Source: CAD feature listing. Evaluate the final solid. Frame: model axes, mm. A direction names the side the tool comes from. Give positions to 0.01 mm unless a question says otherwise; leave off trailing zeros. Loops run counter-clockwise (first coordinate to the right, second up) from the corner with the lowest first, then second, coordinate; pieces in that order, holes last. Notation, with made-up numbers: M -30.5,62.25 L -13.5,62.25 A35 cw -13.5,97.25 Z; hole C 67,14 d10. An arc over 180 degrees is marked long. Answer in a Markdown table with one row per item.
```python
from build123d import *

# Parameters (mm, degrees)
CROQUIS1_R              = 1.000000216
CROQUIS1_R_2            = 1.000000063
CROQUIS1_R_3            = 1.000000073
CROQUIS1_R_4            = 0.999999979
CROQUIS1_R_5            = 1.000000424
CROQUIS1_R_6            = 1.000000593
CROQUIS1_W              = 42
CROQUIS1_H              = 20
SALIENTE_EXTRUIR1_DEPTH = 5.5
CROQUIS2_W              = 16.5
CROQUIS2_H              = 2.5
SALIENTE_EXTRUIR2_DEPTH = 0.5
CROQUIS3_W              = 16.5
CROQUIS3_H              = 20
CORTAR_EXTRUIR1_DEPTH   = 2.5
REDONDEO1_R             = 3


with BuildPart() as part:
    # Croquis1 → Saliente-Extruir1 (new body)
    with BuildSketch(Plane(origin=(0, 0, 0), x_dir=(1, 0, 0), z_dir=(0, 1, 0))):
        with BuildLine():
            Line((-35.503347099, 12.623865495), (-35.503347099, 5.124115358))
            Line((-35.503347099, 5.124115358), (-25.50434655, 7.623865495))
            Line((-25.50434655, 7.623865495), (-25.50434655, -7.376134505))
            Line((-25.50434655, -7.376134505), (-35.503347099, -4.876384368))
            Line((-35.503347099, -4.876384368), (-35.503347099, -12.376134505))
            Line((-35.503347099, -12.376134505), (-19.003347099, -12.376134505))
            Line((-19.003347099, -12.376134505), (-12.8396222, -15.276134123))
            Line((-12.8396222, -15.276134123), (34.184025109, -15.270214667))
            ThreePointArc((34.184025109, -15.270214667), (36.167856769, -14.448338396), (36.98973304, -12.464506735))
            Line((36.98973304, -12.464506735), (36.98973304, 12.712237726))
            ThreePointArc((36.98973304, 12.712237726), (36.167960213, 14.69617283), (34.184025109, 15.517945657))
            Line((34.184025109, 15.517945657), (-12.8396222, 15.523865114))
            Line((-12.8396222, 15.523865114), (-19.003347099, 12.623865495))
            Line((-19.003347099, 12.623865495), (-35.503347099, 12.623865495))
        make_face()
        with Locations((-22.254346372, 6.123865279)):
            Circle(CROQUIS1_R, mode=Mode.SUBTRACT)
        with Locations((-15.504346839, 5.123865558)):
            Circle(CROQUIS1_R_2, mode=Mode.SUBTRACT)
        with Locations((33.495653377, 5.123865568)):
            Circle(CROQUIS1_R_3, mode=Mode.SUBTRACT)
        with Locations((33.4956531, -4.876133997)):
            Circle(CROQUIS1_R_4, mode=Mode.SUBTRACT)
        with Locations((-15.504347678, -4.876134927)):
            Circle(CROQUIS1_R_5, mode=Mode.SUBTRACT)
        with Locations((-22.254345484, -5.876135091)):
            Circle(CROQUIS1_R_6, mode=Mode.SUBTRACT)
        with Locations((8.99565345, 0.123865495)):
            Rectangle(CROQUIS1_W, CROQUIS1_H, mode=Mode.SUBTRACT)
    extrude(amount=SALIENTE_EXTRUIR1_DEPTH)

    # Croquis2 → Saliente-Extruir2 (add)
    with BuildSketch(Plane(origin=(0, 5.5, 0), x_dir=(1, 0, 0), z_dir=(0, 1, 0))):
        with Locations((-27.253347099, -11.126134505)):
            Rectangle(CROQUIS2_W, CROQUIS2_H)
        with Locations((-27.253347099, 11.373865495)):
            Rectangle(CROQUIS2_W, CROQUIS2_H)
    extrude(amount=SALIENTE_EXTRUIR2_DEPTH)

    # Croquis3 → Cortar-Extruir1 (cut)
    with BuildSketch(Plane(origin=(0, 5.5, 0), x_dir=(1, 0, 0), z_dir=(0, 1, 0))):
        with Locations((-27.253347099, 0.123865495)):
            Rectangle(CROQUIS3_W, CROQUIS3_H)
    extrude(amount=-CORTAR_EXTRUIR1_DEPTH, mode=Mode.SUBTRACT)

    # Redondeo1
    redondeo1_edges = [part.edges().sort_by_distance(p)[0] for p in [
        (-27.253347099, 0, 12.376134505),
        (-27.253347099, 0, -12.623865495),
    ]]
    fillet(redondeo1_edges, radius=REDONDEO1_R)


solid = part.part
```
Q1. Mould query, pull axis Z, two halves, no side actions, for faces 1 (the flat face through (-27, 6, -11)), 2 (the cylindrical face through (-16.5, 2.7, 4.8)), 3 (the flat face through (-16.4, 2.7, 13.6)). Classes: +Z half, -Z half, draft (parallel to the pull), parting line (faces both ways), or undercut.
Values follow:
| item | result |
|---|---|
| face 1 | draft |
| face 2 | undercut |
| face 3 | +Z half |
Q2. Reachability of faces 4 (the flat face through (9, 3, -10.124)), 5 (the flat face through (-27, 5, 9.876)), 6 (the cylindrical face through (-28.971, 0.855, 11.474)) from +Z, -Z, +X, -X, +Y, -Y: full face, straight path, thin tool, end or side. Return the list, or none.
Values follow:
| item | result |
|---|---|
| face 4 | +Y, -Y |
| face 5 | -X, +Y |
| face 6 | +Z, -X, -Y |
Q3. Contact query for flat-ended pins moving along their axis: pin 1 Ø10 at (x, z) = (28, 10.5) entering from +Y; pin 2 Ø3.5 at (y, z) = (1.5, 0.5) entering from -X; pin 3 Ø3.5 at (x, y) = (-30.5, 4.5) entering from +Z; pin 4 Ø1.2 at (x, z) = (-15.5, 4.88) entering from -Y. Output: stop coordinate, or through.
Values follow:
| item | result |
|---|---|
| pin 1 | y = 5.5 |
| pin 2 | x = -25.5 |
| pin 3 | z = 12.38 |
| pin 4 | through |
Q4. Ray query, probe 1 along Z at (x, y) = (26, 0.95); probe 2 along X at (y, z) = (1.95, 2); probe 3 along X at (y, z) = (3.9, -5). Return the intervals inside material, ascending. Write a range as from..to.
Values follow:
| item | result |
|---|---|
| probe 1 | -15.52..-10.12, 9.88..15.27 |
| probe 2 | -25.5..-12, 30..36.99 |
| probe 3 | -19..-16.5, -14.51..-12, 30..32.5, 34.49..36.99 |
Q5. Section query C-C (x = -10). Output: boundary loops of the cut face in (y, z).
Values follow:
| item | result |
|---|---|
| outline | M 0,-15.52 L 5.5,-15.52 L 5.5,-10.12 L 0,-10.12 Z; M 0,9.88 L 5.5,9.88 L 5.5,15.28 L 0,15.28 Z |
Q6. Section query B-B (y = 3.8). Output: boundary loops of the cut face in (x, z).
Values follow:
| item | result |
|---|---|
| outline | M -35.5,-12.62 L -19,-12.62 L -12.84,-15.52 L 34.18,-15.52 A2.81 ccw 36.99,-12.71 L 36.99,12.46 A2.81 ccw 34.18,15.27 L -12.84,15.28 L -19,12.38 L -35.5,12.38 L -35.5,9.88 L -19,9.88 L -19,-10.12 L -35.5,-10.12 Z; hole C -15.5,-5.12 d2; hole C -15.5,4.88 d2; hole M -12,-10.12 L 30,-10.12 L 30,9.88 L -12,9.88 Z; hole C 33.5,-5.12 d2; hole C 33.5,4.88 d2 |
Q7. Section query D-D (x = -2). Output: boundary loops of the cut face in (y, z), plus the area to 3 significant figures.
Values follow:
| item | result |
|---|---|
| outline | M 0,-15.52 L 5.5,-15.52 L 5.5,-10.12 L 0,-10.12 Z; M 0,9.88 L 5.5,9.88 L 5.5,15.27 L 0,15.27 Z |
| area | 59.4 mm^2 |
Q8. Section query A-A (z = -0.5). Output: boundary loops of the cut face in (x, y).
Values follow:
| item | result |
|---|---|
| outline | M -25.5,0 L -12,0 L -12,5.5 L -19,5.5 L -19,3 L -25.5,3 Z; M 30,0 L 36.99,0 L 36.99,5.5 L 30,5.5 Z |
